from build123d import *

# Parameters (mm, degrees)
F0_R     = 2
F1_DEPTH = 3
F3_SIZE  = 5


with BuildPart() as f1:
    # F0 (on Front) → F1 (new body)
    with BuildSketch(Plane.XZ):
        Polygon((-35.7739527003, 50), (-55.7739527003, 50), (-55.7739527003, 0), (-5.7739527003, 0), (-5.7739527003, 20), (-35.7739527003, 20), align=None)
        with Locations((-43.7739527003, 12)):
            Circle(F0_R, mode=Mode.SUBTRACT)
        with Locations((-16.6526697576, 12)):
            Circle(F0_R, mode=Mode.SUBTRACT)
        with Locations((-43.7739527003, 38.9910824597)):
            Circle(F0_R, mode=Mode.SUBTRACT)
    extrude(amount=F1_DEPTH)

    # F2: F1 across face


with BuildPart() as f1_1:
    add(f1.part)
    add(f1.part.mirror(Plane(origin=(-30.7739527003, -1.5, 0), x_dir=(1, 0, 0), z_dir=(0, 0, -1))))

    # F3
    f3_edges = [f1_1.edges().sort_by_distance(p)[0] for p in [
        (-5.773953, -1.5, 20),
        (-5.773953, -1.5, -20),
        (-35.773953, -1.5, 50),
        (-35.773953, -1.5, -50),
        (-55.773953, -1.5, 50),
        (-55.773953, -1.5, -50),
    ]]
    chamfer(f3_edges, length=F3_SIZE)


solid = f1_1.part
Source: CAD feature listing. Evaluate the final solid. Frame: model axes, mm. A direction names the side the tool comes from. Round coordinates to 2 decimals unless told otherwise and drop trailing zeros. Write each loop counter-clockwise with the first axis right and the second up, starting at its lowest first coordinate (ties: lowest second). Pieces come first, ordered by that corner, then holes. Notation, with made-up numbers: M -1,58.25 L 13,58.25 A23 cw 13,74.25 Z; hole C 87,15.25 d8. An arc over 180 degrees is marked long. One line per item, written item: value. Start each with the question number.
Item 1: Ray query, L1, parallel to X at y = -1.2, z = -12; L2, parallel to X at y = -2.55, z = 13; L3, parallel to X at y = -0.15, z = -39. Return the intervals inside material, ascending. Write a range as from..to.
Item 2: Section query A-A (z = 12). Return the cut outline in (x, y), plus the area to 3 significant figures.
Item 3: Section query B-B (y = -2.25). Return the cut outline in (x, z).
Item 4: Section query D-D (z = -27). Return the cut outline in (x, y).
Item 5: Section query C-C (x = -24.5). Return the cut outline in (y, z), plus the area to 3 significant figures.
Item 6: Pin query (flat end, axial travel): pin 1 (0.9 mm diameter, centred on x = -27.5, y = -1, fed in from +Z); pin 2 (1.5 mm diameter, centred on x = -30.5, y = -0.5, fed in from -Z). Return the tip coordinate at first contact, or that it passes through.
Item 7: Mould query, pull axis X, two halves, no side actions, for faces 3 (the flat face through (-23, -1, 20)), 4 (the flat face through (-35.774, -1, 32)), 5 (the cylindrical face through (-45.2, -1.5, 13.4)). Classes: pulls with the +X half, pulls with the -X half, needs draft (parallel to the pull), parting line crosses it, or undercut.
Item 8: Set-up query: faces 1 (the flat face through (-23, -1, -20)), 2 (the flat face through (-46, -1, 50)). Return all of +Z, -Z, +X, -X, +Y, -Y with unobstructed straight access to the full face (end or side cutting, diameter ignored); none if empty.
Result set:
1. L1: x = -55.77..-45.77, -41.77..-18.65, -14.65..-5.77
1. L2: x = -55.77..-45.51, -42.04..-18.38, -14.92..-5.77
1. L3: x = -55.77..-45.77, -41.77..-35.77
2. outline: M -55.77,-3 L -45.77,-3 L -45.77,0 L -55.77,0 Z; M -41.77,-3 L -18.65,-3 L -18.65,0 L -41.77,0 Z; M -14.65,-3 L -5.77,-3 L -5.77,0 L -14.65,0 Z
2. area: 126 mm²
3. outline: M -55.77,-45 L -50.77,-50 L -40.77,-50 L -35.77,-45 L -35.77,-20 L -10.77,-20 L -5.77,-15 L -5.77,15 L -10.77,20 L -35.77,20 L -35.77,45 L -40.77,50 L -50.77,50 L -55.77,45 Z; hole C -43.77,-38.99 d4; hole C -43.77,-12 d4; hole C -43.77,12 d4; hole C -43.77,38.99 d4; hole C -16.65,-12 d4; hole C -16.65,12 d4
4. outline: M -55.77,-3 L -35.77,-3 L -35.77,0 L -55.77,0 Z
5. outline: M -3,-20 L 0,-20 L 0,20 L -3,20 Z
5. area: 120 mm²
6. pin 1: stops at z = 20
6. pin 2: stops at z = -20
7. face 3: needs draft
7. face 4: pulls with the +X half
7. face 5: undercut
8. face 1: -Z, +X, +Y, -Y
8. face 2: +Z, +X, -X, +Y, -Y
